Could you check a few things on this drawing? It's one solid part, dimensions in mm from its lowest x, y, z. A direction names the side the tool comes from. Round coordinates to 2 decimals unless told otherwise and drop trailing zeros. Write each loop counter-clockwise with the first axis right and the second up, starting at its lowest first coordinate (ties: lowest second). Pieces come first, ordered by that corner, then holes. Notation, with made-up numbers: (23.5, -8.5) -> (70.5, -8.5) arc R7 ccw to (70.5, -3.5) -> close; hole circle Ø10 at (63.25, 57). An arc over 180 degrees is marked (long way). Return JSON: item names as keys, results as strings.
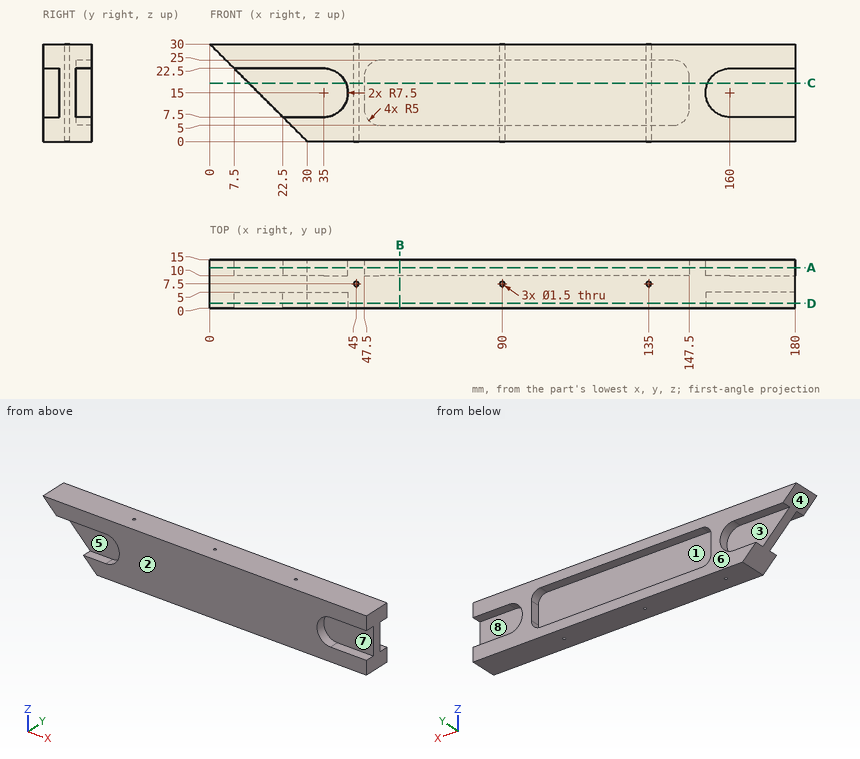
1) For the marked faces 5, 6, 7 and 8, which set-ups out of +Z, -Z, +X, -X, +Y, -Y let a thin tool reach every point of the face, with its end or its side?
Return value:
{"face 5": "-X, -Y", "face 6": "+Z, -Z, +X, -X, +Y", "face 7": "+X, -Y", "face 8": "+X, +Y"}
2) I want a section at C-C, the plane z = 18. Please give me the cut outline in (x, y), and give its area (3 significant figures).
Return value:
{"outline": "(12, 5) -> (41.87, 5) -> (41.87, 0) -> (153.13, 0) -> (153.13, 5) -> (180, 5) -> (180, 10) -> (153.13, 10) -> (153.13, 15) -> (147.5, 15) -> (147.5, 10) -> (47.5, 10) -> (47.5, 15) -> (41.87, 15) -> (41.87, 10) -> (12, 10) -> close; hole circle Ø1.5 at (45, 7.5); hole circle Ø1.5 at (90, 7.5); hole circle Ø1.5 at (135, 7.5)", "area": "1,450 mm²"}
3) If I drill on probe 1 along Y at (x, z) = (45, 7); probe 2 along Y at (x, z) = (135, 22.75); probe 3 along Z at (x, y) = (163, 13.5), over which ranges is the centre line in solid material (lowest first)? Write a range as [from, to].
Return value:
{"probe 1": "[0, 6.75], [8.25, 15]", "probe 2": "[0, 6.75], [8.25, 10]", "probe 3": "[0, 7.5], [22.5, 30]"}
4) Will these pins go through, and if not, where does the flat tip stop? pin 1 Ø4 at (x, y) = (167, 11.5) entering from -Z; pin 2 Ø12 at (x, z) = (28.5, 14.5) entering from -Y; pin 3 Ø4 at (x, z) = (134.5, 15) entering from +Y; pin 4 Ø5.5 at (y, z) = (13, 13.5) entering from +X.
Return value:
{"pin 1": "z = 0", "pin 2": "y = 5", "pin 3": "y = 10", "pin 4": "x = 153.82"}
5) I want a section at A-A, the plane y = 12.5. Please give me the cut outline in (x, z).
Return value:
{"outline": "(0, 30) -> (7.5, 22.5) -> (35, 22.5) arc R7.5 cw to (35, 7.5) -> (22.5, 7.5) -> (30, 0) -> (180, 0) -> (180, 7.5) -> (160, 7.5) arc R7.5 cw to (160, 22.5) -> (180, 22.5) -> (180, 30) -> close; hole (47.5, 10) arc R5 ccw to (52.5, 5) -> (142.5, 5) arc R5 ccw to (147.5, 10) -> (147.5, 20) arc R5 ccw to (142.5, 25) -> (52.5, 25) arc R5 ccw to (47.5, 20) -> close"}
6) I want a section at B-B, the plane x = 58.5. Please give me the cut outline in (y, z), and give its area (3 significant figures).
Return value:
{"outline": "(0, 0) -> (15, 0) -> (15, 5) -> (10, 5) -> (10, 25) -> (15, 25) -> (15, 30) -> (0, 30) -> close", "area": "350 mm²"}
7) I want a section at D-D, the plane y = 1.5. Please give me the cut outline in (x, z).
Return value:
{"outline": "(0, 30) -> (7.5, 22.5) -> (35, 22.5) arc R7.5 cw to (35, 7.5) -> (22.5, 7.5) -> (30, 0) -> (180, 0) -> (180, 7.5) -> (160, 7.5) arc R7.5 cw to (160, 22.5) -> (180, 22.5) -> (180, 30) -> close"}
8) Thinking about a two-plate mould opening in Z: for the marked faces 1, 2, 3 and 4, which applies, pulls with the +Z half, pulls with the -Z half, needs draft (parallel to the pull), parting line crosses it, or undercut?
Return value:
{"face 1": "undercut", "face 2": "needs draft", "face 3": "undercut", "face 4": "pulls with the -Z half"}
